Model file for the job. Use its own axes, mm. A direction names the side the tool comes from. Coordinates: 2 decimals unless noted, no trailing zeros. Write each loop counter-clockwise with the first axis right and the second up, starting at its lowest first coordinate (ties: lowest second). Pieces come first, ordered by that corner, then holes. Notation, with made-up numbers: M 51,-10.75 L 104,-10.75 A19 cw 104,16.25 Z; hole C -7,89 d10. An arc over 180 degrees is marked long. Put each result on its own line as item: value. Start each with the question number.
Q1. Cut at A-A (z = 78.5). Write the cut outline in (x, y), then the cut area to 3 significant figures.
Q2. Drill centre lines: line 1 along X through (y, z) = (4.65, -80); line 2 along Z through (x, y) = (-69.5, 3.75); line 3 along X through (y, z) = (4.75, -50). Where is each one in solid material? Low to high.
Q3. Which spindle directions (+Z, -Z, +X, -X, +Y, -Y) get a long thin tool onto all of the face, cutting with end or side? Do faces 1 (the flat face through (-94, 3, -55)), 2 (the flat face through (85, 3, -100)), 3 (the flat face through (55, 3, 94)), 4 (the flat face through (70, 3, -97)), 5 (the flat face through (100, 3, 85)). Say none if no direction does.
Q4. Pull direction Z, two halves, no side cores. Call faces 6 (the flat face through (100, 3, 1)), 7 (the flat face through (106, 3, -55)), 8 (the flat face through (103, 3, -70)): pulls with the +Z half, pulls with the -Z half, needs draft (parallel to the pull), parting line crosses it, or undercut.
Q5. Cut at B-B (x = 61.5). Write the cut outline in (y, z).
Q6. Drop flat-ended pins along their axis: pin 1 (3 mm diameter, centred on x = 102.5, y = 2.5, fed in from +Z); pin 2 (1.8 mm diameter, centred on y = 2.5, z = -96.5, fed in from +X); pin 3 (1 mm diameter, centred on x = 8.5, z = -75.5, fed in from -Y). Give the stop position or say it passes through.
```python
from build123d import *

# Parameters (mm, degrees)
RESSALTO_EXTRUS_O1_DEPTH = 6
ESBO_O2_W                = 30
ESBO_O2_H                = 6
ESBO_O2_W_2              = 6
ESBO_O2_H_2              = 30
CORTE_EXTRUS_O1_DEPTH    = 10


with BuildPart() as part:
    # Esboço1 → Ressalto-extrusão1 (new body)
    with BuildSketch(Plane(origin=(0, 0, 0), x_dir=(1, 0, 0), z_dir=(0, 1, 0))):
        Polygon((100, 70), (100, 100), (-100, 100), (-100, -100), (100, -100), (100, -70), (106, -70), (106, -40), (100, -40), (100, 40), (106, 40), (106, 70), align=None)
    extrude(amount=RESSALTO_EXTRUS_O1_DEPTH)

    # Esboço2 → Corte-extrusão1 (cut)
    with BuildSketch(Plane(origin=(0, 6, 0), x_dir=(1, 0, 0), z_dir=(0, 1, 0))):
        with Locations((-55, -97)):
            Rectangle(ESBO_O2_W, ESBO_O2_H)
        with Locations((55, -97)):
            Rectangle(ESBO_O2_W, ESBO_O2_H)
        with Locations((-55, 97)):
            Rectangle(ESBO_O2_W, ESBO_O2_H)
        with Locations((55, 97)):
            Rectangle(ESBO_O2_W, ESBO_O2_H)
        with Locations((-97, 55)):
            Rectangle(ESBO_O2_W_2, ESBO_O2_H_2)
        with Locations((-97, -55)):
            Rectangle(ESBO_O2_W_2, ESBO_O2_H_2)
    extrude(amount=-CORTE_EXTRUS_O1_DEPTH, mode=Mode.SUBTRACT)


solid = part.part
```
Computed values:
1. outline: M -100,0 L 100,0 L 100,6 L -100,6 Z
1. area: 1,200 mm2
2. line 1: -100 to 100
2. line 2: -94 to 94
2. line 3: -94 to 106
3. face 1: -X, +Y, -Y
3. face 2: -Z, +X, -X, +Y, -Y
3. face 3: +Z, +Y, -Y
3. face 4: -Z, +Y, -Y
3. face 5: +Z, +X, +Y, -Y
4. face 6: undercut
4. face 7: needs draft
4. face 8: pulls with the -Z half
5. outline: M 0,-94 L 6,-94 L 6,94 L 0,94 Z
6. pin 1: z = 70
6. pin 2: x = 100
6. pin 3: y = 0
